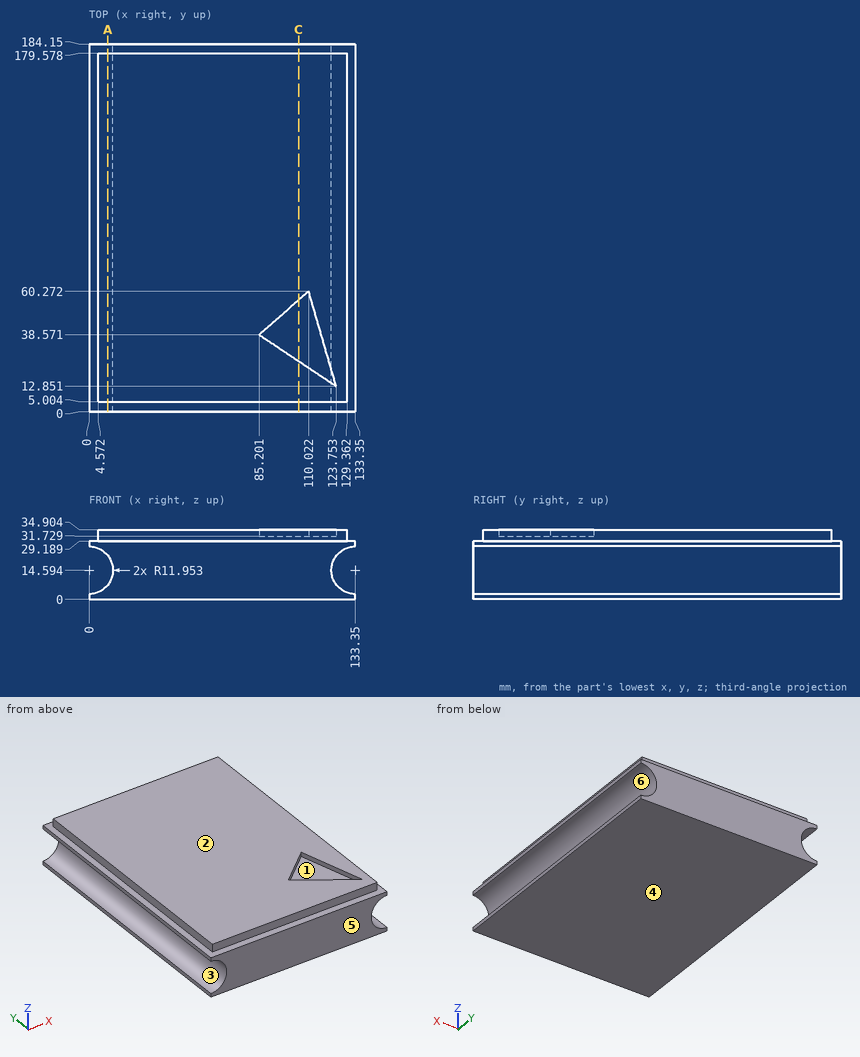
Verification items for this drawing (mm, ordinates from the low corner). A direction names the side the tool comes from. Give positions to 0.01 mm unless a question says otherwise; leave off trailing zeros. Loops run counter-clockwise (first coordinate to the right, second up) from the corner with the lowest first, then second, coordinate; pieces in that order, holes last.
(1) Thickness scan on L1, parallel to X at y = 97, z = 33.5; L2, parallel to Z at x = 112, y = 37; L3, parallel to Z at x = 7.5, y = 155 (1 decimal). Record the ranges inside material, lowest first.
From the geometry:
L1: x = 4.57 to 129.36
L2: z = 0 to 31.73
L3: z = 0 to 5.3, 23.9 to 34.9
(2) Depth check by flat-ended pin: pin 1 Ø6.5 at (y, z) = (96.5, 32.5) entering from +X; pin 2 Ø8 at (x, y) = (110, 37.5) entering from +Z; pin 3 Ø4.5 at (x, z) = (50, 32.5) entering from -Y. Enter the tip coordinate at first touch or a pass-through.
From the geometry:
pin 1: stops at x = 129.36
pin 2: stops at z = 31.73
pin 3: stops at y = 5
(3) Section check C-C on x = 105. Record the cut outline in (y, z), then the cut area to 3 significant figures.
From the geometry:
outline: (0, 0) - (184.15, 0) - (184.15, 29.19) - (179.58, 29.19) - (179.58, 34.9) - (55.88, 34.9) - (55.88, 31.73) - (25.36, 31.73) - (25.36, 34.9) - (5, 34.9) - (5, 29.19) - (0, 29.19) - close
area: 6,280 mm2
(4) Set-up check for the marked faces 1 and 2: record each of +Z, -Z, +X, -X, +Y, -Y from which the full face is reachable in a straight line by a thin tool's end or side.
From the geometry:
face 1: +Z
face 2: +Z, +X, -X, +Y, -Y
(5) Release check for a two-part mould opening along Z. For the marked faces 3, 4, 5 and 6 record: released by +Z, released by -Z, zero draft, split by the parting line, or undercut.
From the geometry:
face 3: undercut
face 4: released by -Z
face 5: zero draft
face 6: undercut
(6) Section check A-A on x = 9.5. Record the cut outline in (y, z), then the cut area to 3 significant figures.
From the geometry:
outline: (0, 0) - (184.15, 0) - (184.15, 7.34) - (0, 7.34) - close; (0, 21.85) - (184.15, 21.85) - (184.15, 29.19) - (179.58, 29.19) - (179.58, 34.9) - (5, 34.9) - (5, 29.19) - (0, 29.19) - close
area: 3,700 mm2
